from build123d import *

# Parameters (mm, degrees)
SKETCH1_W           = 20
SKETCH1_H           = 200
SKETCH1_H_2         = 10
SKETCH1_W_2         = 14.875
BOSS_EXTRUDE1_DEPTH = 10


with BuildPart() as part:
    # Sketch1 → Boss-Extrude1 (new body)
    with BuildSketch(Plane.XY):
        with Locations((0, -115)):
            Rectangle(SKETCH1_W, SKETCH1_H)
        with Locations((0, -10)):
            Rectangle(SKETCH1_W, SKETCH1_H_2)
        Polygon((-10, 5), (-10, -5), (10, -5), (10, 5), (5.773502692, 5), (2.886751346, 0), (-2.886751346, 0), (-5.773502692, 5), align=None)
        with Locations((-17.4375, 0)):
            Rectangle(SKETCH1_W_2, SKETCH1_H_2)
        with Locations((17.4375, 0)):
            Rectangle(SKETCH1_W_2, SKETCH1_H_2)
    extrude(amount=BOSS_EXTRUDE1_DEPTH)


solid = part.part
Build history of the part. All positions in model axes, mm. A direction names the side the tool comes from. Round coordinates to 2 decimals unless told otherwise and drop trailing zeros. Write each loop counter-clockwise with the first axis right and the second up, starting at its lowest first coordinate (ties: lowest second). Pieces come first, ordered by that corner, then holes. Notation, with made-up numbers: (28.25, -1) - (69.25, -1) arc R22 ccw to (69.25, 26) - close; hole circle Ø7 at (87, 4.5). An arc over 180 degrees is marked (long way). One line per question, with ' | ' between items.
1. Drop flat-ended pins along their axis: pin 1 Ø1.7 at (x, z) = (-1, 5.5) entering from +Y; pin 2 Ø3 at (y, z) = (-181.5, 6.5) entering from +X; pin 3 Ø1 at (y, z) = (-34, 4) entering from -X. Give the stop position or say it passes through.
Results are:
pin 1: y = 0 | pin 2: x = 10 | pin 3: x = -10
2. Band-saw the part on B-B, the plane x = 19. Write the cut outline in (y, z).
Results are:
outline: (-5, 0) - (5, 0) - (5, 10) - (-5, 10) - close
3. Band-saw the part on C-C, the plane y = -42.5. Write the cut outline in (x, z).
Results are:
outline: (-10, 0) - (10, 0) - (10, 10) - (-10, 10) - close
4. Mould opens along X. For faces 6 (the face through (0, -215, 5)), 7 (the face through (-4.31, 2.465, 4.93)), 8 (the face through (24.875, 0, 5)) say: released by +X, released by -X, zero draft, split by the parting line, or undercut.
Results are:
face 6: zero draft | face 7: undercut | face 8: released by +X
5. Drill centre lines: line 1 along X through (y, z) = (-44, 2.25); line 2 along Y through (x, z) = (20, 7); line 3 along Y through (x, z) = (4, 8). Where is each one in solid material? Low to high. Write a range as from..to.
Results are:
line 1: -10..10 | line 2: -5..5 | line 3: -215..1.93
6. Band-saw the part on A-A, the plane z = 8. Write the cut outline in (x, y) (1 decimal).
Results are:
outline: (-24.9, -5) - (-10, -5) - (-10, -215) - (10, -215) - (10, -5) - (24.9, -5) - (24.9, 5) - (5.8, 5) - (2.9, 0) - (-2.9, 0) - (-5.8, 5) - (-24.9, 5) - close
7. Tool access for faces 1 (the face through (4.35, 2.535, 4.93)), 2 (the face through (17, -5, 5)), 3 (the face through (-10, -109, 5)), 4 (the face through (-4, -96, 0)), 5 (the face through (-15, 5, 5)): list every direction of +Z, -Z, +X, -X, +Y, -Y with a clear straight run to the whole face (end or side of a thin tool).
Results are:
face 1: +Z, -Z, +Y | face 2: +Z, -Z, +X, -Y | face 3: +Z, -Z, -X, -Y | face 4: -Z, +X, -X, +Y, -Y | face 5: +Z, -Z, +X, -X, +Y
